Could you check a few things on this model? Use its own coordinates, in mm. A direction names the side the tool comes from. Coordinates: 2 decimals unless noted, no trailing zeros. Order: outer loops, then holes, each group sorted by start corner. A loop starts at its lowest first (then second) coordinate and runs counter-clockwise, first axis right, second up.
```python
from build123d import *

# Parameters (mm, degrees)
F0_R     = 10.5
F0_R_2   = 5
F0_R_3   = 1.8
F1_DEPTH = 4
F2_DEPTH = 14


with BuildPart() as f1:
    # F0 (on Top) → F1 (new body)
    with BuildSketch(Plane.XY):
        Circle(F0_R)
        Circle(F0_R_2, mode=Mode.SUBTRACT)
        Circle(F0_R_2)
        with BuildLine():
            ThreePointArc((3.039737, 2.6), (4, 0), (3.039737, -2.6))
            Line((3.039737, -2.6), (-3.039737, -2.6))
            ThreePointArc((-3.039737, -2.6), (-4, 0), (-3.039737, 2.6))
            Line((-3.039737, 2.6), (3.039737, 2.6))
        make_face(mode=Mode.SUBTRACT)
        with BuildLine():
            Line((-3.039737, -2.6), (3.039737, -2.6))
            ThreePointArc((3.039737, -2.6), (4, 0), (3.039737, 2.6))
            Line((3.039737, 2.6), (-3.039737, 2.6))
            ThreePointArc((-3.039737, 2.6), (-4, 0), (-3.039737, -2.6))
        make_face()
        Circle(F0_R_3, mode=Mode.SUBTRACT)
    extrude(amount=F1_DEPTH)

    # F0 (on Top) → F2 (join)
    with BuildSketch(Plane.XY):
        Circle(F0_R_2)
        with BuildLine():
            ThreePointArc((3.039737, 2.6), (4, 0), (3.039737, -2.6))
            Line((3.039737, -2.6), (-3.039737, -2.6))
            ThreePointArc((-3.039737, -2.6), (-4, 0), (-3.039737, 2.6))
            Line((-3.039737, 2.6), (3.039737, 2.6))
        make_face(mode=Mode.SUBTRACT)
    extrude(amount=F2_DEPTH)


solid = f1.part
```
Item 1: Suppose I cut it at B-B (y = 0). List the corners of the cut face in (x, z) for me, and give its area (3 significant figures).
Item 2: For pin 1 Ø3 at (x, y) = (0, 0) entering from +Z; pin 2 Ø6 at (x, z) = (-5, 1.5) entering from +Y; pin 3 Ø4 at (x, z) = (3, 2) entering from -Y; pin 4 Ø4 at (x, z) = (-3.5, 12) entering from -Y, each with a flat end and sliding along its axis, tell me the tip position at first contact or that it passes through.
Item 3: Suppose I cut it at C-C (z = 9.75). List the corners of the cut face in (x, y) for me, and give its area (3 significant figures).
Item 4: Which directions (+Z, -Z, +X, -X, +Y, -Y) give clear straight access to the entire face, cutting with the end or side of a thin tool? Please do faces 4 (the face through (0, -2.6, 9)), 5 (the face through (0, -3, 14)).
Item 5: Suppose I cut it at D-D (y = -4.5). List the corners of the cut face in (x, z) for me.
Item 6: Thinking about a two-plate mould opening in X: for faces 1 (the face through (1.717, 0.541, 1.972)), 2 (the face through (10, 3.2, 2)), 3 (the face through (2, 0, 0)), which applies, +X half, -X half, draft (parallel to the pull), parting line (faces both ways), or undercut?
Item 7: Suppose I cut it at A-A (x = 0). List the corners of the cut face in (y, z) for me.
Item 8: I need wall thicknesses on line 1 (Y direction, x = 0, z = 2.5); line 2 (Z direction, x = 3.5, y = -7); line 3 (X direction, y = 0.5, z = 9.5). Which ranges of each line are inside material? Lowest first, please.
Geometry results:
1. outline: (-10.5, 0) - (-1.8, 0) - (-1.8, 4) - (-4, 4) - (-4, 14) - (-5, 14) - (-5, 4) - (-10.5, 4) - close; (1.8, 0) - (10.5, 0) - (10.5, 4) - (5, 4) - (5, 14) - (4, 14) - (4, 4) - (1.8, 4) - close
1. area: 89.6 mm2
2. pin 1: passes through
2. pin 2: stops at y = 10.31
2. pin 3: stops at y = -10.45
2. pin 4: stops at y = -4.77
3. outline: circle Ø10 at (0, 0); hole (-3.04, -2.6) - (3.04, -2.6) arc R4 ccw to (3.04, 2.6) - (-3.04, 2.6) arc R4 ccw to start
3. area: 40.1 mm2
4. face 4: +Z
4. face 5: +Z, +X, -X, +Y, -Y
5. outline: (-9.49, 0) - (9.49, 0) - (9.49, 4) - (2.18, 4) - (2.18, 14) - (-2.18, 14) - (-2.18, 4) - (-9.49, 4) - close
6. face 1: undercut
6. face 2: parting line
6. face 3: draft
7. outline: (-10.5, 0) - (-1.8, 0) - (-1.8, 4) - (-2.6, 4) - (-2.6, 14) - (-5, 14) - (-5, 4) - (-10.5, 4) - close; (1.8, 0) - (10.5, 0) - (10.5, 4) - (5, 4) - (5, 14) - (2.6, 14) - (2.6, 4) - (1.8, 4) - close
8. line 1: y = -10.5 to -1.8, 1.8 to 10.5
8. line 2: z = 0 to 4
8. line 3: x = -4.97 to -3.97, 3.97 to 4.97
